Geometry: final body of the model. Coordinates: model frame, mm. A direction names the side the tool comes from. Round coordinates to 2 decimals unless told otherwise and drop trailing zeros. Loops run counter-clockwise (first coordinate to the right, second up) from the corner with the lowest first, then second, coordinate; pieces in that order, holes last. Notation, with made-up numbers: (68, 54) - (121, 54) arc R19 cw to (121, 64) - close; hole circle Ø1 at (-20, -18). An arc over 180 degrees is marked (long way). Answer in a Markdown table with one row per item. Add a question column.
from build123d import *

# Parameters (mm, degrees)
EXTRUDE_1_DEPTH     = 45
SKETCH_2_R          = 7.5
CUT_EXTRUDE_2_DEPTH = 24
SKETCH_3_W          = 32
SKETCH_3_H          = 20
EXTRUDE_4_DEPTH     = 24
SKETCH_4_R          = 8
CUT_EXTRUDE_3_DEPTH = 24


with BuildPart() as part:
    # 草图1 → 凸台-拉伸1 (new body)
    with BuildSketch(Plane.XY):
        Polygon((-11.5, -5), (11.5, -5), (11.5, 5), (16, 5), (16, 13), (-16, 13), (-16, 5), (-11.5, 5), align=None)
    extrude(amount=-EXTRUDE_1_DEPTH)

    # 草图2 → 切除-拉伸2 (cut)
    with BuildSketch(Plane(origin=(0, 13, 0), x_dir=(1, 0, 0), z_dir=(0, 1, 0))):
        with Locations(Location((0, 12.5, 0), (0, 0, 270))):
            Circle(SKETCH_2_R)
    extrude(amount=-CUT_EXTRUDE_2_DEPTH, mode=Mode.SUBTRACT)

    # 草图3 → 凸台-拉伸4 (add)
    with BuildSketch(Plane(origin=(0, 13, 0), x_dir=(1, 0, 0), z_dir=(0, 1, 0))):
        with Locations((0, 35)):
            Rectangle(SKETCH_3_W, SKETCH_3_H)
    extrude(amount=EXTRUDE_4_DEPTH)

    # 草图4 → 切除-拉伸3 (cut)
    with BuildSketch(Plane.XY.offset(-25)):
        with Locations((0, 37)):
            Circle(SKETCH_4_R)
    extrude(amount=-CUT_EXTRUDE_3_DEPTH, mode=Mode.SUBTRACT)


solid = part.part
1) Section C-C, the plane z = -12.5. Return the cut outline in (x, y), and give its area (3 significant figures).
2) Reachability of faces 4 (the flat face through (11.5, 0, -22)), 5 (the flat face through (-11.5, 0, -22)), 6 (the flat face through (7.3, 13, -9.5)), 7 (the flat face through (12, 37, -35)), 8 (the cylindrical face through (0, 29, -35)) from +Z, -Z, +X, -X, +Y, -Y: full face, straight path, thin tool, end or side. Return the list, or none.
3) Contact query for flat-ended pins moving along their axis: pin 1 Ø1.3 at (x, z) = (13, -27.5) entering from -Y; pin 2 Ø5 at (y, z) = (-0.5, -28) entering from -X; pin 3 Ø12.5 at (x, z) = (-2.5, -11.5) entering from +Y. Output: stop coordinate, or through.
4) Pull-direction query (X, two-part tool) for faces 1 (the cylindrical face through (0, 4, -20)), 2 (the flat face through (16, 17, -32)), 3 (the flat face through (0, 25, -25)); classes: pulls with the +X half, pulls with the -X half, needs draft (parallel to the pull), parting line crosses it, or undercut.
5) Section D-D, the plane y = 34.5. Return the cut outline in (x, z), and give its area (3 significant figures).
6) Section A-A, the plane x = 0. Return the cut outline in (y, z).
7) Material intervals for line 1 along X through (y, z) = (0.5, -12.5); line 2 along X through (y, z) = (8.5, -12.5); line 3 along Y through (x, z) = (14, -3.5), sorted ascending. Write a range as from..to.
8) Section B-B, the plane y = 11. Return the cut outline in (x, z).
Evaluation:
| question | item | result |
|---|---|---|
| 1 | outline | (-16, 5) - (-11.5, 5) - (-11.5, -5) - (-7.5, -5) - (-7.5, 13) - (-16, 13) - close; (7.5, -5) - (11.5, -5) - (11.5, 5) - (16, 5) - (16, 13) - (7.5, 13) - close |
| 1 | area | 216 mm² |
| 2 | face 4 | +Z, -Z, +X, -Y |
| 2 | face 5 | +Z, -Z, -X, -Y |
| 2 | face 6 | +Z, +X, -X, +Y |
| 2 | face 7 | +Z, -Z, +X, -X, +Y |
| 2 | face 8 | +Z, -Z, +Y |
| 3 | pin 1 | stops at y = 5 |
| 3 | pin 2 | stops at x = -11.5 |
| 3 | pin 3 | stops at y = 13 |
| 4 | face 1 | undercut |
| 4 | face 2 | pulls with the +X half |
| 4 | face 3 | needs draft |
| 5 | outline | (-16, -45) - (-7.6, -45) - (-7.6, -25) - (-16, -25) - close; (7.6, -45) - (16, -45) - (16, -25) - (7.6, -25) - close |
| 5 | area | 336 mm² |
| 6 | outline | (-5, -45) - (29, -45) - (29, -25) - (13, -25) - (13, -20) - (-5, -20) - close; (-5, -5) - (13, -5) - (13, 0) - (-5, 0) - close |
| 7 | line 1 | x = -11.5..-7.5, 7.5..11.5 |
| 7 | line 2 | x = -16..-7.5, 7.5..16 |
| 7 | line 3 | y = 5..13 |
| 8 | outline | (-16, -45) - (16, -45) - (16, 0) - (-16, 0) - close; hole circle Ø15 at (0, -12.5) |
